For this review, use the dimensioned drawing (mm, ordinates from the lowest corner) and the shaded views. Give positions to 0.01 mm unless a question says otherwise; leave off trailing zeros. Order: outer loops, then holes, each group sorted by start corner. A loop starts at its lowest first (then second) coordinate and runs counter-clockwise, first axis right, second up. Notation, with made-up numbers: M 29.25,62.25 L 74.25,62.25 A12 cw 74.25,72.25 Z; hole C 82.5,32.5 d10. An arc over 180 degrees is marked long. Answer as CSV lines item,"result". Start each with the question number.
1. We need section B-B, the plane y = 8.75. Give the boundary of the cut face in (x, z) (1 decimal), and give its area (3 significant figures).
2. We need section D-D, the plane x = 117.5. Give the boundary of the cut face in (y, z) (1 decimal).
3. We need section C-C, the plane z = 36. Give the boundary of the cut face in (x, y).
4. We need section A-A, the plane x = 11. Give the boundary of the cut face in (y, z) (1 decimal).
5. For line 1 along Z through (x, y) = (135.5, 6.75) (1 decimal); line 2 along Z through (x, y) = (138.5, 9) (1 decimal); line 3 along Z through (x, y) = (98, 1.5) (1 decimal), list the stretches that pass through material, from the lowest coordinate up.
6. Clearance check with a flat-ended pin moving along its axis: P1, Ø6, axis at y = 1.5, z = 77, coming from the +X side. State where the tip first meets the part, or that it passes through.
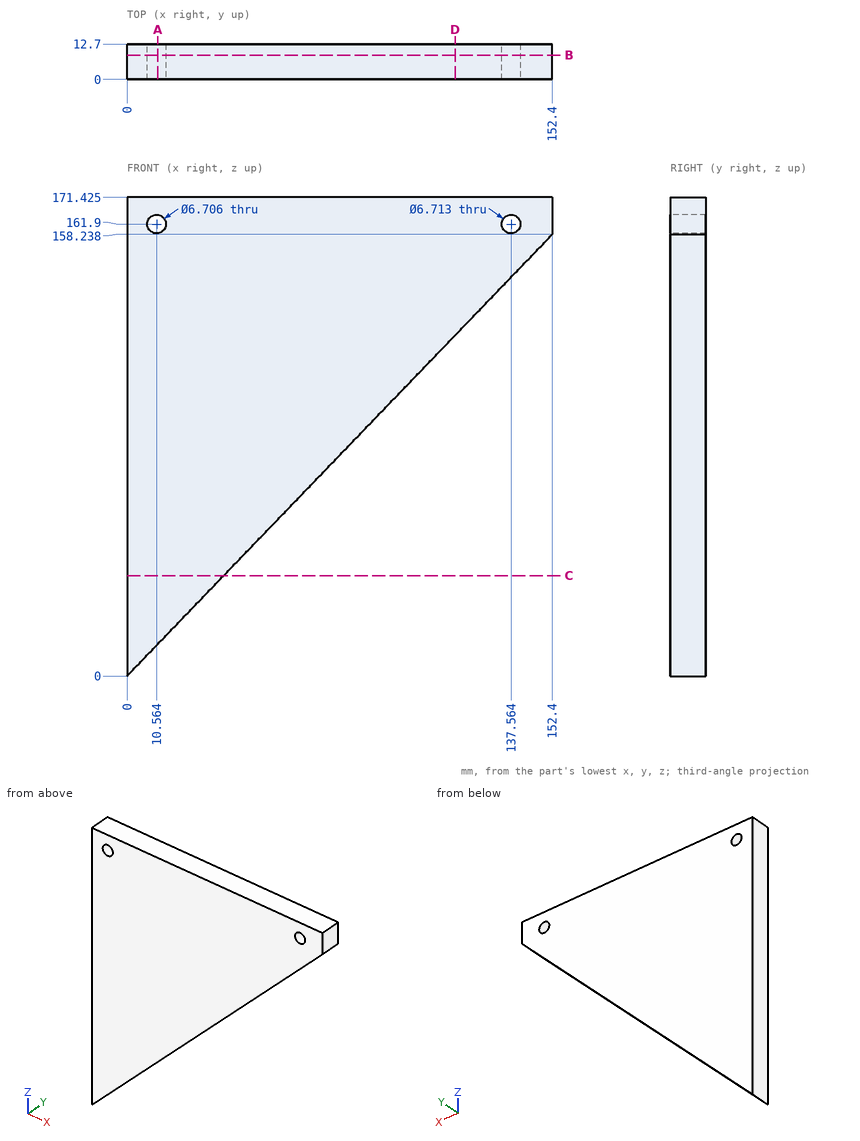
Result set:
1,outline,"M 0,0 L 152.4,158.2 L 152.4,171.4 L 0,171.4 Z; hole C 10.6,161.9 d6.7; hole C 137.6,161.9 d6.7"
1,area,"14,000 mm2"
2,outline,"M 0,122 L 12.7,122 L 12.7,171.4 L 0,171.4 Z"
3,outline,"M 0,0 L 34.67,0 L 34.67,12.7 L 0,12.7 Z"
4,outline,"M 0,11.4 L 12.7,11.4 L 12.7,158.6 L 0,158.6 Z; M 0,165.2 L 12.7,165.2 L 12.7,171.4 L 0,171.4 Z"
5,line 1,"140.7 to 159.3, 164.5 to 171.4"
5,line 2,"143.8 to 158.7, 165.1 to 171.4"
5,line 3,"101.8 to 171.4"
6,P1,"x = 77.05"
